```python
from build123d import *

# Parameters (mm, degrees)
SKETCH1_W           = 130
SKETCH1_H           = 89.679378249
SKETCH1_R           = 2.25
SKETCH1_W_2         = 71.3
SKETCH1_H_2         = 79
BOSS_EXTRUDE1_DEPTH = 5
FILLET1_R           = 3
SKETCH2_R           = 5
CUT_EXTRUDE1_DEPTH  = 5
SKETCH3_R           = 2.25
CUT_EXTRUDE2_DEPTH  = 5


with BuildPart() as part:
    # Sketch1 → Boss-Extrude1 (new body)
    with BuildSketch(Plane.XY):
        with Locations((65, -44.839689125)):
            Rectangle(SKETCH1_W, SKETCH1_H)
        with Locations((125, -5)):
            Circle(SKETCH1_R, mode=Mode.SUBTRACT)
        with Locations((125, -55)):
            Circle(SKETCH1_R, mode=Mode.SUBTRACT)
        with Locations((5, -55)):
            Circle(SKETCH1_R, mode=Mode.SUBTRACT)
        with Locations((5, -5)):
            Circle(SKETCH1_R, mode=Mode.SUBTRACT)
        with Locations((62.35, -44.179378249)):
            Rectangle(SKETCH1_W_2, SKETCH1_H_2, mode=Mode.SUBTRACT)
    extrude(amount=BOSS_EXTRUDE1_DEPTH)

    # Fillet1
    fillet1_edges = [part.edges().sort_by_distance(p)[0] for p in [
        (0, 0, 2.5),
        (130, 0, 2.5),
        (130, -89.679378249, 2.5),
        (0, -89.679378249, 2.5),
    ]]
    fillet(fillet1_edges, radius=FILLET1_R)

    # Sketch2 → Cut-Extrude1 (cut)
    with BuildSketch(Plane(origin=(0, 0, 0), x_dir=(-1, 0, 0), z_dir=(0, 0, -1))):
        with Locations((-115, -30)):
            Circle(SKETCH2_R)
    extrude(amount=-CUT_EXTRUDE1_DEPTH, mode=Mode.SUBTRACT)

    # Sketch3 → Cut-Extrude2 (cut)
    with BuildSketch(Plane.XY.offset(5)):
        with Locations((125, -42.5)):
            Circle(SKETCH3_R)
        with Locations((125, -17.5)):
            Circle(SKETCH3_R)
    extrude(amount=-CUT_EXTRUDE2_DEPTH, mode=Mode.SUBTRACT)


solid = part.part
```
Input: part model. Units: mm. Frame: model coordinates. A direction names the side the tool comes from. Round coordinates to 2 decimals unless told otherwise and drop trailing zeros. Loops run counter-clockwise (first coordinate to the right, second up) from the corner with the lowest first, then second, coordinate; pieces in that order, holes last. Notation, with made-up numbers: M 12,80 L 39,80 A15 cw 39,104 Z; hole C -2,22.25 d11. An arc over 180 degrees is marked long. Answer in a Markdown table with one row per item. Add a question column.
1. Section C-C (y = -63). Output: boundary loops of the cut face in (x, z), and give its area (4 significant figures).
2. Mould query, pull axis Y, two halves, no side actions, for faces 3 (the face through (127.08, -18.36, 2.54)), 4 (the face through (129.1, -0.86, 2.54)), 5 (the face through (0, -45, 2)). Classes: released by +Y, released by -Y, zero draft, split by the parting line, or undercut.
3. Ray query, probe 1 along Y at (x, z) = (125, 2.35); probe 2 along Y at (x, z) = (5, 1.4); probe 3 along Y at (x, z) = (40.5, 0.75). Return the intervals inside material, ascending.
4. Section D-D (z = 1.3). Give the number of separate pieces and of enclosed holes in the cut face, and give its area (3 significant figures).
5. Section A-A (x = 65). Output: boundary loops of the cut face in (y, z), and give its area (3 significant figures).
6. Section B-B (y = -42.5). Output: boundary loops of the cut face in (x, z), and give its area (3 significant figures).
7. Set-up query: faces 1 (the face through (129.1, -88.82, 2.54)), 2 (the face through (98, -45, 2)). Return all of +Z, -Z, +X, -X, +Y, -Y with unobstructed straight access to the full face (end or side cutting, diameter ignored); none if empty.
Values follow:
| question | item | result |
|---|---|---|
| 1 | outline | M 0,0 L 26.7,0 L 26.7,5 L 0,5 Z; M 98,0 L 130,0 L 130,5 L 98,5 Z |
| 1 | area | 293.5 mm^2 |
| 2 | face 3 | undercut |
| 2 | face 4 | released by +Y |
| 2 | face 5 | zero draft |
| 3 | probe 1 | -89.68 to -57.25, -52.75 to -44.75, -40.25 to -19.75, -15.25 to -7.25, -2.75 to 0 |
| 3 | probe 2 | -89.68 to -57.25, -52.75 to -7.25, -2.75 to 0 |
| 3 | probe 3 | -89.68 to -83.68, -4.68 to 0 |
| 4 | separate pieces | 1 |
| 4 | enclosed holes | 8 |
| 4 | area | 5,840 mm^2 |
| 5 | outline | M -89.68,0 L -83.68,0 L -83.68,5 L -89.68,5 Z; M -4.68,0 L 0,0 L 0,5 L -4.68,5 Z |
| 5 | area | 53.4 mm^2 |
| 6 | outline | M 0,0 L 26.7,0 L 26.7,5 L 0,5 Z; M 98,0 L 122.75,0 L 122.75,5 L 98,5 Z; M 127.25,0 L 130,0 L 130,5 L 127.25,5 Z |
| 6 | area | 271 mm^2 |
| 7 | face 1 | +Z, -Z, +X, -Y |
| 7 | face 2 | +Z, -Z |
